The model under review builds one solid part; all positions refer to its coordinate system, in mm. A direction names the side the tool comes from. Round coordinates to 2 decimals unless told otherwise and drop trailing zeros. Loops run counter-clockwise (first coordinate to the right, second up) from the corner with the lowest first, then second, coordinate; pieces in that order, holes last. Notation, with made-up numbers: M 74,-28 L 84,-28 A30 ccw 84,-1 Z; hole C 50.25,-5.5 d2. An arc over 180 degrees is marked long. Answer as a JSON object with one key per item and string values. Group by question number.
Item 1: Consider section C-C (z = -13). Give the boundary of the cut face in (x, y).
Item 2: To check wall thickness, follow line 1 (Z direction, x = -15.25, y = 0.4); line 2 (Y direction, x = -14, z = -1); line 3 (X direction, y = 0.9, z = 15.5). State the ranges of each line that lie inside material, in increasing order.
Item 3: Insertion check: P1, Ø4, axis at x = -15.25, z = 15.25, coming from the +Y side; P2, Ø1.5, axis at x = -6.5, z = -3.5, coming from the -Y side; P3, Ø1.7, axis at x = 9.5, y = 3, coming from the +Z side; P4, Ø1, axis at y = 2.5, z = -1.5, coming from the +X side. Each pin has a flat end and moves straight along its axis. Give the tip position at first contact, or say it passes through.
Item 4: Consider section A-A (x = -15.25). Give the boundary of the cut face in (y, z).
Item 5: Tool access review of faces 5 (the face through (-17.4, 0.86, 17.43)), 6 (the face through (9.6, 2.7, 15)): name each direction out of +Z, -Z, +X, -X, +Y, -Y from which nothing blocks a thin tool from reaching the whole face with its end or side.
Item 6: Consider section B-B (y = 1). Give the boundary of the cut face in (x, z), and give its area (3 significant figures).
Item 7: The part is to be moulded in two halves that separate along X. For faces 1 (the face through (9.6, 2.7, 14.5)), 2 (the face through (17.4, 0.86, -17.43)), 3 (the face through (13.75, 0.86, 15.18)), 4 (the face through (10, 1.85, 17)), say which applies: +X half, -X half, draft (parallel to the pull), parting line (faces both ways), or undercut.
Item 8: Consider section D-D (x = -9.5). Give the boundary of the cut face in (y, z), and give its area (3 significant figures).
```python
from build123d import *

# Parameters (mm, degrees)
SKETCH1_R           = 1.5
BOSS_EXTRUDE1_DEPTH = 1.75
BOSS_EXTRUDE4_DEPTH = 3
BOSS_EXTRUDE5_DEPTH = 0.5
CUT_EXTRUDE1_REACH  = 5.5
SKETCH7_R           = 0.25


with BuildPart() as part:
    # Sketch1 → Boss-Extrude1 (new body)
    with BuildSketch(Plane(origin=(0, 0, 0), x_dir=(1, 0, 0), z_dir=(0, 1, 0))):
        with BuildLine():
            Line((-16, 18), (16, 18))
            ThreePointArc((16, 18), (17.414213562, 17.414213562), (18, 16))
            Line((18, 16), (18, -16))
            ThreePointArc((18, -16), (17.414213562, -17.414213562), (16, -18))
            Line((16, -18), (-16, -18))
            ThreePointArc((-16, -18), (-17.414213562, -17.414213562), (-18, -16))
            Line((-18, -16), (-18, 16))
            ThreePointArc((-18, 16), (-17.414213562, 17.414213562), (-16, 18))
        make_face()
        with Locations((-15.25, 15.25)):
            Circle(SKETCH1_R, mode=Mode.SUBTRACT)
        with Locations((15.25, 15.25)):
            Circle(SKETCH1_R, mode=Mode.SUBTRACT)
        with Locations((15.25, -15.25)):
            Circle(SKETCH1_R, mode=Mode.SUBTRACT)
        with Locations((-15.25, -15.25)):
            Circle(SKETCH1_R, mode=Mode.SUBTRACT)
    extrude(amount=BOSS_EXTRUDE1_DEPTH)

    # Sketch2 → Boss-Extrude4 (add)
    with BuildSketch(Plane.XY.offset(18)):
        with BuildLine():
            Line((7.580760647, 1.75), (11.580760647, 1.75))
            Line((11.580760647, 1.75), (11.580760647, 3.240036049))
            ThreePointArc((11.580760647, 3.240036049), (11.522182003, 3.381457405), (11.380760647, 3.440036049))
            Line((11.380760647, 3.440036049), (10.607400333, 3.440036049))
            ThreePointArc((10.607400333, 3.440036049), (10.465978977, 3.498614693), (10.407400333, 3.640036049))
            Line((10.407400333, 3.640036049), (10.407400333, 3.917594602))
            ThreePointArc((10.407400333, 3.917594602), (10.348821689, 4.059015958), (10.207400333, 4.117594602))
            Line((10.207400333, 4.117594602), (8.648098096, 4.117594602))
            ThreePointArc((8.648098096, 4.117594602), (8.50667674, 4.059015958), (8.448098096, 3.917594602))
            Line((8.448098096, 3.917594602), (8.448098096, 3.640036049))
            ThreePointArc((8.448098096, 3.640036049), (8.389519452, 3.498614693), (8.248098096, 3.440036049))
            Line((8.248098096, 3.440036049), (7.780760647, 3.440036049))
            ThreePointArc((7.780760647, 3.440036049), (7.63933929, 3.381457405), (7.580760647, 3.240036049))
            Line((7.580760647, 3.240036049), (7.580760647, 1.75))
        make_face()
        with BuildLine():
            Line((8.648098096, 4.017594602), (10.207400333, 4.017594602))
            ThreePointArc((10.207400333, 4.017594602), (10.278111011, 3.98830528), (10.307400333, 3.917594602))
            Line((10.307400333, 3.917594602), (10.307400333, 3.640036049))
            ThreePointArc((10.307400333, 3.640036049), (10.395268299, 3.427904014), (10.607400333, 3.340036049))
            Line((10.607400333, 3.340036049), (11.380760647, 3.340036049))
            ThreePointArc((11.380760647, 3.340036049), (11.451471325, 3.310746727), (11.480760647, 3.240036049))
            Line((11.480760647, 3.240036049), (11.480760647, 1.85))
            Line((11.480760647, 1.85), (7.680760647, 1.85))
            Line((7.680760647, 1.85), (7.680760647, 3.240036049))
            ThreePointArc((7.680760647, 3.240036049), (7.710049968, 3.310746727), (7.780760647, 3.340036049))
            Line((7.780760647, 3.340036049), (8.248098096, 3.340036049))
            ThreePointArc((8.248098096, 3.340036049), (8.460230131, 3.427904014), (8.548098096, 3.640036049))
            Line((8.548098096, 3.640036049), (8.548098096, 3.917594602))
            ThreePointArc((8.548098096, 3.917594602), (8.577387418, 3.98830528), (8.648098096, 4.017594602))
        make_face(mode=Mode.SUBTRACT)
    extrude(amount=-BOSS_EXTRUDE4_DEPTH)

    # Sketch5 → Boss-Extrude5 (add)
    with BuildSketch(Plane(origin=(0, 0, 15), x_dir=(-1, 0, 0), z_dir=(0, 0, -1))):
        with BuildLine():
            Line((-7.580760647, 1.75), (-7.580760647, 3.240036049))
            ThreePointArc((-7.580760647, 3.240036049), (-7.63933929, 3.381457405), (-7.780760647, 3.440036049))
            Line((-7.780760647, 3.440036049), (-8.248098096, 3.440036049))
            ThreePointArc((-8.248098096, 3.440036049), (-8.389519452, 3.498614693), (-8.448098096, 3.640036049))
            Line((-8.448098096, 3.640036049), (-8.448098096, 3.917594602))
            ThreePointArc((-8.448098096, 3.917594602), (-8.50667674, 4.059015958), (-8.648098096, 4.117594602))
            Line((-8.648098096, 4.117594602), (-10.207400333, 4.117594602))
            ThreePointArc((-10.207400333, 4.117594602), (-10.348821689, 4.059015958), (-10.407400333, 3.917594602))
            Line((-10.407400333, 3.917594602), (-10.407400333, 3.640036049))
            ThreePointArc((-10.407400333, 3.640036049), (-10.465978977, 3.498614693), (-10.607400333, 3.440036049))
            Line((-10.607400333, 3.440036049), (-11.380760647, 3.440036049))
            ThreePointArc((-11.380760647, 3.440036049), (-11.522182003, 3.381457405), (-11.580760647, 3.240036049))
            Line((-11.580760647, 3.240036049), (-11.580760647, 1.75))
            Line((-11.580760647, 1.75), (-7.580760647, 1.75))
        make_face()
    extrude(amount=BOSS_EXTRUDE5_DEPTH)

    # Sketch7 → Cut-Extrude1 (cut, up to next)
    with BuildSketch(Plane(origin=(0, 0, 14.5), x_dir=(-1, 0, 0), z_dir=(0, 0, -1)), mode=Mode.PRIVATE) as cut_extrude1_sk1:
        with Locations((-10.302378592, 3.199328245)):
            Circle(SKETCH7_R)
    cut_extrude1_tool1 = extrude(cut_extrude1_sk1.sketch, amount=-CUT_EXTRUDE1_REACH, mode=Mode.PRIVATE) & part.part
    add(cut_extrude1_tool1.solids().sort_by_distance((10.302379, 3.199328, 14.5))[0], mode=Mode.SUBTRACT)
    # Sketch7 → Cut-Extrude1 (cut, up to next)
    with BuildSketch(Plane(origin=(0, 0, 14.5), x_dir=(-1, 0, 0), z_dir=(0, 0, -1)), mode=Mode.PRIVATE) as cut_extrude1_sk2:
        with Locations((-9.502378592, 3.199328245)):
            Circle(SKETCH7_R)
    cut_extrude1_tool2 = extrude(cut_extrude1_sk2.sketch, amount=-CUT_EXTRUDE1_REACH, mode=Mode.PRIVATE) & part.part
    add(cut_extrude1_tool2.solids().sort_by_distance((9.502379, 3.199328, 14.5))[0], mode=Mode.SUBTRACT)
    # Sketch7 → Cut-Extrude1 (cut, up to next)
    with BuildSketch(Plane(origin=(0, 0, 14.5), x_dir=(-1, 0, 0), z_dir=(0, 0, -1)), mode=Mode.PRIVATE) as cut_extrude1_sk3:
        with Locations((-8.702378592, 3.199328245)):
            Circle(SKETCH7_R)
    cut_extrude1_tool3 = extrude(cut_extrude1_sk3.sketch, amount=-CUT_EXTRUDE1_REACH, mode=Mode.PRIVATE) & part.part
    add(cut_extrude1_tool3.solids().sort_by_distance((8.702379, 3.199328, 14.5))[0], mode=Mode.SUBTRACT)


solid = part.part
```
Geometry results:
{
 "1": {"outline": "M -18,0 L 18,0 L 18,1.75 L -18,1.75 Z"},
 "2": {"line 1": "z = -18 to -16.75, -13.75 to 13.75, 16.75 to 18", "line 2": "y = 0 to 1.75", "line 3": "x = -18 to -16.73, -13.77 to 13.77, 16.73 to 18"},
 "3": {"P1": "stops at y = 1.75", "P2": "stops at y = 0", "P3": "stops at z = 15", "P4": "passes through"},
 "4": {"outline": "M 0,-18 L 1.75,-18 L 1.75,-16.75 L 0,-16.75 Z; M 0,-13.75 L 1.75,-13.75 L 1.75,13.75 L 0,13.75 Z; M 0,16.75 L 1.75,16.75 L 1.75,18 L 0,18 Z"},
 "5": {"face 5": "+Z, -X, +Y, -Y", "face 6": "+Z"},
 "6": {"outline": "M -18,-16 A2 ccw -16,-18 L 16,-18 A2 ccw 18,-16 L 18,16 A2 ccw 16,18 L -16,18 A2 ccw -18,16 Z; hole C -15.25,-15.25 d3; hole C -15.25,15.25 d3; hole C 15.25,-15.25 d3; hole C 15.25,15.25 d3", "area": "1,260 mm^2"},
 "7": {"face 1": "draft", "face 2": "+X half", "face 3": "undercut", "face 4": "undercut"},
 "8": {"outline": "M 0,-18 L 1.75,-18 L 1.75,18 L 0,18 Z", "area": "63.0 mm^2"}
}
